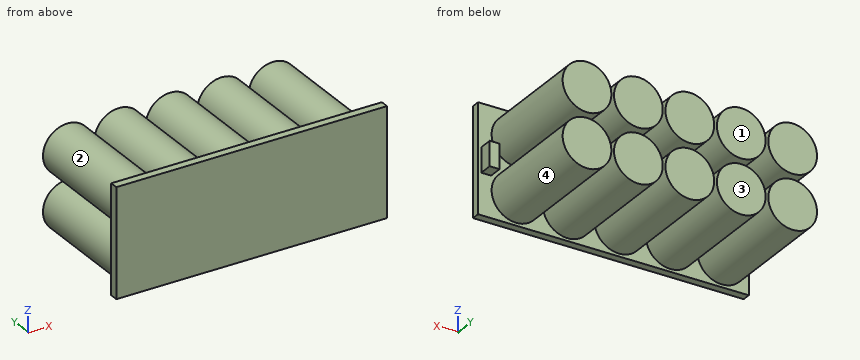
from build123d import *

# Parameters (mm, degrees)
SKETCH_1_W      = 100
SKETCH_1_H      = 40
EXTRUDE_2_DEPTH = 3
SKETCH_2_R      = 9
EXTRUDE_3_DEPTH = 42
SKETCH_3_W      = 3.629615038
SKETCH_3_H      = 9.091657085
EXTRUDE_4_DEPTH = 5


with BuildPart() as part:
    # 草图1 → 凸台-拉伸2 (new body)
    with BuildSketch(Plane(origin=(0, 0, 0), x_dir=(1, 0, 0), z_dir=(0, 1, 0))):
        Rectangle(SKETCH_1_W, SKETCH_1_H)
    extrude(amount=EXTRUDE_2_DEPTH)

    # 草图2 → 凸台-拉伸3 (add)
    with BuildSketch(Plane(origin=(0, 3, 0), x_dir=(1, 0, 0), z_dir=(0, 1, 0))):
        with Locations((-40, -10)):
            Circle(SKETCH_2_R)
        with Locations((-21, -10)):
            Circle(SKETCH_2_R)
        with Locations((-2, -10)):
            Circle(SKETCH_2_R)
        with Locations((17, -10)):
            Circle(SKETCH_2_R)
        with Locations((36, -10)):
            Circle(SKETCH_2_R)
        with Locations((-21, 10)):
            Circle(SKETCH_2_R)
        with Locations((-2, 10)):
            Circle(SKETCH_2_R)
        with Locations((17, 10)):
            Circle(SKETCH_2_R)
        with Locations((36, 10)):
            Circle(SKETCH_2_R)
        with Locations((-40, 10)):
            Circle(SKETCH_2_R)
    extrude(amount=EXTRUDE_3_DEPTH)

    # 草图3 → 凸台-拉伸4 (add)
    with BuildSketch(Plane(origin=(0, 3, 0), x_dir=(1, 0, 0), z_dir=(0, 1, 0))):
        with Locations((46.996489689, 0.280393631)):
            Rectangle(SKETCH_3_W, SKETCH_3_H)
    extrude(amount=EXTRUDE_4_DEPTH)


solid = part.part
Read the model definition and answer for the solid it produces. Units are mm, in the model's axes. Face numbers are marked on the shaded views. A direction names the side the tool comes from. Give positions to 0.01 mm unless a question says otherwise; leave off trailing zeros. Loops run counter-clockwise (first coordinate to the right, second up) from the corner with the lowest first, then second, coordinate; pieces in that order, holes last. Notation, with made-up numbers: (-19, 85.5) -> (14, 85.5) arc R28 cw to (14, 114.5) -> close; hole circle Ø6 at (6.25, 70). An arc over 180 degrees is marked (long way). Use a Markdown table: item, result.
Q1. Each of these flat-tipped pins is pushed along its axis until it touches: pin 1 (5 mm diameter, centred on y = 39, z = -8, fed in from +X); pin 2 (3 mm diameter, centred on x = 48, z = -2.5, fed in from +Y); pin 3 (4 mm diameter, centred on y = 14.5, z = 5.5, fed in from +X). Where does it stop, or does it pass through?
Solved:
| item | result |
|---|---|
| pin 1 | stops at x = 45 |
| pin 2 | stops at y = 8 |
| pin 3 | stops at x = 44.65 |
Q2. Find the intervals of material crossed by line 1 along X through (y, z) = (10, 4); line 2 along X through (y, z) = (16, 8); line 3 along X through (y, z) = (6.5, 4), in increasing order.
Solved:
| item | result |
|---|---|
| line 1 | x = -46.71 to -33.29, -27.71 to -14.29, -8.71 to 4.71, 10.29 to 23.71, 29.29 to 42.71 |
| line 2 | x = -48.77 to -31.23, -29.77 to -12.23, -10.77 to 6.77, 8.23 to 25.77, 27.23 to 44.77 |
| line 3 | x = -46.71 to -33.29, -27.71 to -14.29, -8.71 to 4.71, 10.29 to 23.71, 29.29 to 42.71, 45.18 to 48.81 |
Q3. Section B-B, the plane x = -2 is taken. Determine the outline of the cut face in (y, z).
Solved:
| item | result |
|---|---|
| outline | (0, -20) -> (3, -20) -> (3, -19) -> (45, -19) -> (45, -1) -> (3, -1) -> (3, 1) -> (45, 1) -> (45, 19) -> (3, 19) -> (3, 20) -> (0, 20) -> close |
Q4. Section D-D, the plane x = 13 is taken. Determine the outline of the cut face in (y, z), then the cut area to 3 significant figures.
Solved:
| item | result |
|---|---|
| outline | (0, -20) -> (3, -20) -> (3, -18.06) -> (45, -18.06) -> (45, -1.94) -> (3, -1.94) -> (3, 1.94) -> (45, 1.94) -> (45, 18.06) -> (3, 18.06) -> (3, 20) -> (0, 20) -> close |
| area | 1,470 mm^2 |
Q5. Section C-C, the plane z = 10 is taken. Determine the outline of the cut face in (x, y).
Solved:
| item | result |
|---|---|
| outline | (-50, 0) -> (50, 0) -> (50, 3) -> (45, 3) -> (45, 45) -> (27, 45) -> (27, 3) -> (26, 3) -> (26, 45) -> (8, 45) -> (8, 3) -> (7, 3) -> (7, 45) -> (-11, 45) -> (-11, 3) -> (-12, 3) -> (-12, 45) -> (-30, 45) -> (-30, 3) -> (-31, 3) -> (-31, 45) -> (-49, 45) -> (-49, 3) -> (-50, 3) -> close |
Q6. Determine the mould class of the marked faces 3 and 4 for opening direction X: pulls with the +X half, pulls with the -X half, needs draft (parallel to the pull), parting line crosses it, or undercut.
Solved:
| item | result |
|---|---|
| face 3 | needs draft |
| face 4 | undercut |
Q7. Section A-A, the plane y = 21 is taken. Count the separate pieces of the cut face and the enclosed holes in it, then the cut area to 3 significant figures.
Solved:
| item | result |
|---|---|
| separate pieces | 10 |
| enclosed holes | 0 |
| area | 2,540 mm^2 |
Q8. A tool of negligible diameter and unlimited length cuts with its end or side. For the marked faces 1 and 2, from which of +Z, -Z, +X, -X, +Y, -Y can it reach the whole face along a straight path? Write none if from no direction.
Solved:
| item | result |
|---|---|
| face 1 | +Z, -Z, +X, -X, +Y |
| face 2 | +Y |
